```python
from build123d import *

# Parameters (mm, degrees)
BOSS_EXTRUDE1_DEPTH = 25
SKETCH3_W           = 72
SKETCH3_H           = 90
BOSS_EXTRUDE2_DEPTH = 25
SKETCH4_W           = 37.059895825
SKETCH4_H           = 5.488186397
CUT_EXTRUDE1_DEPTH  = 50
BOSS_EXTRUDE3_DEPTH = 15


with BuildPart() as part:
    # Sketch2 → Boss-Extrude1 (new body)
    with BuildSketch(Plane(origin=(0, 0, 0), x_dir=(1, 0, 0), z_dir=(0, 1, 0))):
        with BuildLine():
            Line((0, 0), (62.597938144, 0))
            Line((62.597938144, 0), (125.195876289, 0))
            Line((125.195876289, 0), (125.195876289, 24))
            Line((125.195876289, 24), (74.474226804, 24))
            ThreePointArc((74.474226804, 24), (62.474226804, 36), (74.474226804, 48))
            Line((74.474226804, 48), (125.195876289, 48))
            Line((125.195876289, 48), (125.195876289, 72))
            Line((125.195876289, 72), (0, 72))
            Line((0, 72), (0, 0))
        make_face()
    extrude(amount=BOSS_EXTRUDE1_DEPTH)

    # Sketch3 → Boss-Extrude2 (add)
    with BuildSketch(Plane.ZY):
        with Locations((-36, 45)):
            Rectangle(SKETCH3_W, SKETCH3_H)
    extrude(amount=BOSS_EXTRUDE2_DEPTH)

    # Sketch4 → Cut-Extrude1 (cut)
    with BuildSketch(Plane.XY):
        with Locations((-6.470052088, 2.744093199)):
            Rectangle(SKETCH4_W, SKETCH4_H)
    extrude(amount=-CUT_EXTRUDE1_DEPTH, mode=Mode.SUBTRACT)

    # Sketch5 → Boss-Extrude3 (add)
    with BuildSketch(Plane.ZY.offset(25)):
        with BuildLine():
            Line((0, 5.488186397), (-50, 5.488186397))
            Line((-50, 5.488186397), (-50, 0))
            Line((-50, 0), (-72, 0))
            Line((-72, 0), (-72, 30.033370453))
            Line((-72, 30.033370453), (-62, 30.033370453))
            ThreePointArc((-62, 30.033370453), (-36, 15), (-10, 30.033370453))
            Line((-10, 30.033370453), (0, 30.033370453))
            Line((0, 30.033370453), (0, 5.488186397))
        make_face()
        with BuildLine():
            Line((-50, 90), (0, 90))
            Line((0, 90), (0, 84.511813603))
            Line((0, 84.511813603), (0, 59.966629547))
            Line((0, 59.966629547), (-10, 59.966629547))
            ThreePointArc((-10, 59.966629547), (-36, 75), (-62, 59.966629547))
            Line((-62, 59.966629547), (-72, 59.966629547))
            Line((-72, 59.966629547), (-72, 90))
            Line((-72, 90), (-50, 90))
        make_face()
    extrude(amount=BOSS_EXTRUDE3_DEPTH)


solid = part.part
```
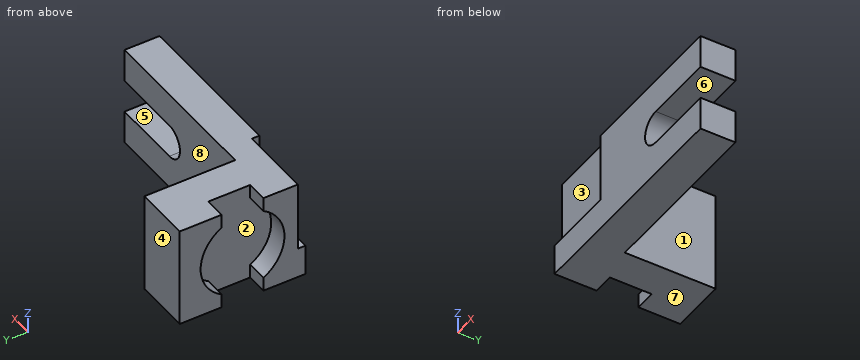
For this review, take the finished solid that the model builds, in its own axes (mm). Face numbers are marked on the shaded views. A direction names the side the tool comes from. Give positions to 0.01 mm unless a question says otherwise; leave off trailing zeros. Write each loop counter-clockwise with the first axis right and the second up, starting at its lowest first coordinate (ties: lowest second). Pieces come first, ordered by that corner, then holes.
Item 1: Wall thickness on probe 1 along Y at (x, z) = (14.5, -9.5); probe 2 along X at (y, z) = (28.5, -10); probe 3 along Y at (x, z) = (11.5, -11.5): over which ranges is each line inside the solid? List them lowest first.
Item 2: Machinability: for the marked faces 1, 2, 3, 4 and 5, which of the approach directions +Z, -Z, +X, -X, +Y, -Y give a long, thin tool a straight path to every point of the face, cutting with its end or side? Answer none if there is none.
Item 3: Insertion check: P1, Ø4, axis at y = 42.5, z = -34.5, coming from the -X side; P2, Ø19.5, axis at y = 45.5, z = -18, coming from the +X side; P3, Ø4.5, axis at y = 2, z = -36, coming from the -X side. Each pin has a flat end and moves straight along its axis. Give the tip position at first contact, or say it passes through.
Item 4: Take a section at C-C (z = -36). Give the boundary of the cut face in (x, y), and give its area (3 significant figures).
Item 5: Take a section at B-B (y = 27). Give the boundary of the cut face in (x, z), and give its area (3 significant figures).
Item 6: Take a section at A-A (x = -27). Give the boundary of the cut face in (y, z).
Item 7: Take a section at D-D (x = 33.5). Give the boundary of the cut face in (y, z).
Item 8: The part is to be moulded in two halves that separate along Z. For the marked faces 6, 7 and 8, say which applies: +Z half, -Z half, draft (parallel to the pull), parting line (faces both ways), or undercut.
Established:
1. probe 1: y = 0 to 25
1. probe 2: x = -40 to 0
1. probe 3: y = 5.49 to 25
2. face 1: +Z, -Z, +X, +Y
2. face 2: -X
2. face 3: +Z, -X, -Y
2. face 4: +Z, -Z, +X, -X, +Y
2. face 5: +X, +Y, -Y
3. P1: stops at x = -25
3. P2: stops at x = 0
3. P3: stops at x = 12.06
4. outline: (-40, 5.49) - (12.06, 5.49) - (12.06, 0) - (62.47, 0) - (62.47, 25) - (0, 25) - (0, 90) - (-40, 90) - (-40, 75) - (-25, 75) - (-25, 15) - (-40, 15) - close
4. area: 3,980 mm2
5. outline: (-40, -72) - (0, -72) - (0, 0) - (-40, 0) - (-40, -12) - (-25, -12) - (-25, -60) - (-40, -60) - close
5. area: 2,160 mm2
6. outline: (0, -72) - (30.03, -72) - (30.03, -62) arc R30 cw to (30.03, -10) - (30.03, 0) - (5.49, 0) - (5.49, -50) - (0, -50) - close; (59.97, -72) - (90, -72) - (90, 0) - (59.97, 0) - (59.97, -10) arc R30 cw to (59.97, -62) - close
7. outline: (0, -72) - (25, -72) - (25, 0) - (0, 0) - close
8. face 6: undercut
8. face 7: -Z half
8. face 8: draft
